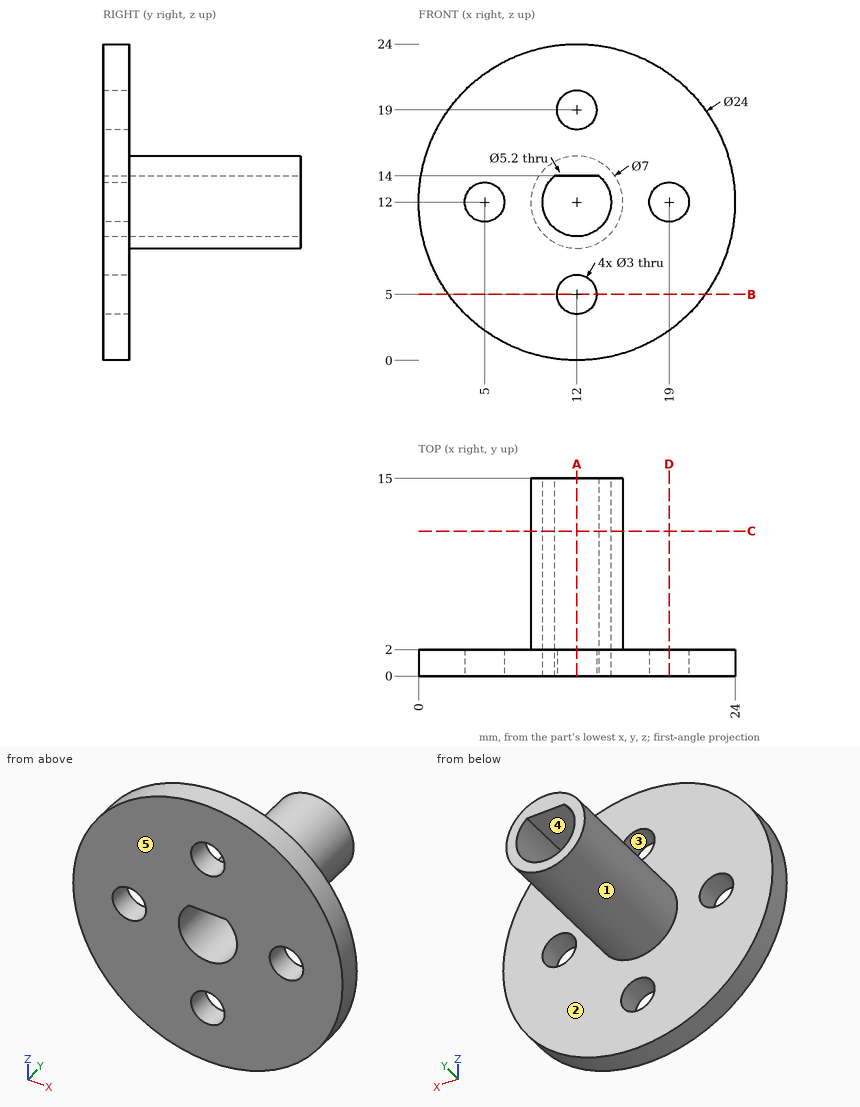
Can you work these out from the drawing? Everything is in mm from the part's minimum corner. A direction names the side the tool comes from. Round coordinates to 2 decimals unless told otherwise and drop trailing zeros. Loops run counter-clockwise (first coordinate to the right, second up) from the corner with the lowest first, then second, coordinate; pieces in that order, holes last. Notation, with made-up numbers: (31, -4.75) -> (48, -4.75) arc R21 ccw to (48, 25.25) -> close; hole circle Ø11 at (13.5, 44.5). An arc over 180 degrees is marked (long way). Answer in a Markdown table with one row per item.
Item 1: If I drill on probe 1 along X at (y, z) = (1.55, 12); probe 2 along Z at (x, y) = (11, 1.5); probe 3 along X at (y, z) = (4, 12), over which ranges is the centre line in solid material (lowest first)?
Answer block:
| item | result |
|---|---|
| probe 1 | 0 to 3.5, 6.5 to 9.4, 14.6 to 17.5, 20.5 to 24 |
| probe 2 | 0.04 to 3.88, 6.12 to 9.6, 14 to 17.88, 20.12 to 23.96 |
| probe 3 | 8.5 to 9.4, 14.6 to 15.5 |
Item 2: Suppose I cut it at B-B, the plane z = 5. List the corners of the cut face in (x, y) for me.
Answer block:
| item | result |
|---|---|
| outline | (2.25, 0) -> (10.5, 0) -> (10.5, 2) -> (2.25, 2) -> close; (13.5, 0) -> (21.75, 0) -> (21.75, 2) -> (13.5, 2) -> close |
Item 3: Suppose I cut it at C-C, the plane y = 11. List the corners of the cut face in (x, z) for me, plus the area to 3 significant figures.
Answer block:
| item | result |
|---|---|
| outline | circle Ø7 at (12, 12); hole (10.34, 14) arc R2.6 ccw (long way) to (13.66, 14) -> close |
| area | 18.6 mm² |
Item 4: We'd pull the mould along Z, two halves only. Please class the marked faces 1, 2 and 3: released by +Z, released by -Z, zero draft, split by the parting line, or undercut.
Answer block:
| item | result |
|---|---|
| face 1 | split by the parting line |
| face 2 | zero draft |
| face 3 | undercut |
Item 5: On a 3-axis mill with a long thin cutter (end or side, diameter ignored), from which of +Z, -Z, +X, -X, +Y, -Y can I reach the whole of each face in a straight line? I mean the marked faces 4 and 5. Say none if no direction works.
Answer block:
| item | result |
|---|---|
| face 4 | +Y, -Y |
| face 5 | +Z, -Z, +X, -X, -Y |
Item 6: Suppose I cut it at A-A, the plane x = 12. List the corners of the cut face in (y, z) for me.
Answer block:
| item | result |
|---|---|
| outline | (0, 0) -> (2, 0) -> (2, 3.5) -> (0, 3.5) -> close; (0, 6.5) -> (2, 6.5) -> (2, 8.5) -> (15, 8.5) -> (15, 9.4) -> (0, 9.4) -> close; (0, 14) -> (15, 14) -> (15, 15.5) -> (2, 15.5) -> (2, 17.5) -> (0, 17.5) -> close; (0, 20.5) -> (2, 20.5) -> (2, 24) -> (0, 24) -> close |
Item 7: Suppose I cut it at D-D, the plane x = 19. List the corners of the cut face in (y, z) for me, plus the area to 3 significant figures.
Answer block:
| item | result |
|---|---|
| outline | (0, 2.25) -> (2, 2.25) -> (2, 10.5) -> (0, 10.5) -> close; (0, 13.5) -> (2, 13.5) -> (2, 21.75) -> (0, 21.75) -> close |
| area | 33.0 mm² |
Item 8: Will these pins go through, and if not, where does the flat tip stop? P1, Ø1.5, axis at x = 15, y = 8, coming from the +Z side; P2, Ø4, axis at x = 19, z = 12, coming from the +Y side; P3, Ø1, axis at x = 12, y = 10, coming from the -Z side; P4, Ø1.8, axis at x = 12, z = 19, coming from the -Y side.
Answer block:
| item | result |
|---|---|
| P1 | z = 14.68 |
| P2 | y = 2 |
| P3 | z = 8.5 |
| P4 | through |
